from build123d import *

# Parameters (mm, degrees)
SKETCH1_R           = 1.016
SKETCH1_R_2         = 1.397
BOSS_EXTRUDE1_DEPTH = 3.175


with BuildPart() as part:
    # Sketch1 → Boss-Extrude1 (new body)
    with BuildSketch(Plane.XZ.offset(3.175)):
        with BuildLine():
            Line((12.7, 38.1), (6.35, 38.1))
            ThreePointArc((6.35, 38.1), (-7.120384182, 32.520384182), (-12.7, 19.05))
            Line((-12.7, 19.05), (-12.7, -38.1))
            Line((-12.7, -38.1), (12.7, -38.1))
            Line((12.7, -38.1), (12.7, 38.1))
        make_face()
        with Locations(Location((5.08, 20.828, 0), (0, 0, 90))):  # turned: the seam where the file's is
            Circle(SKETCH1_R, mode=Mode.SUBTRACT)
        with Locations(Location((-5.08, 20.828, 0), (0, 0, 90))):  # turned: the seam where the file's is
            Circle(SKETCH1_R, mode=Mode.SUBTRACT)
        with Locations(Location((-5.08, -27.792, 0), (0, 0, 90))):  # turned: the seam where the file's is
            Circle(SKETCH1_R, mode=Mode.SUBTRACT)
        with Locations(Location((5.08, -27.792, 0), (0, 0, 90))):  # turned: the seam where the file's is
            Circle(SKETCH1_R, mode=Mode.SUBTRACT)
        with Locations(Location((0, 31.75, 0), (0, 0, 90))):  # turned: the seam where the file's is
            Circle(SKETCH1_R_2, mode=Mode.SUBTRACT)
        Polygon((3.65, 17.018), (10, 17.018), (10, -23.982), (-10, -23.982), (-10, 17.018), (-3.65, 17.018), (-3.65, 20.193), (3.65, 20.193), align=None, mode=Mode.SUBTRACT)
    extrude(amount=-BOSS_EXTRUDE1_DEPTH)


solid = part.part
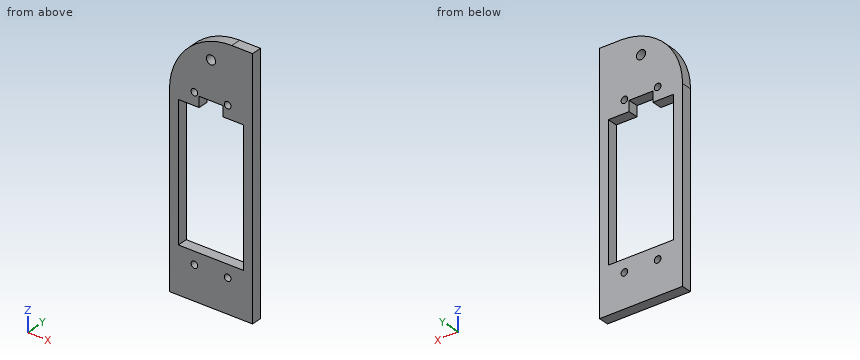
CAD build for the part. Positions are in the model's coordinates, mm. Round coordinates to 2 decimals unless told otherwise and drop trailing zeros. Write each loop counter-clockwise with the first axis right and the second up, starting at its lowest first coordinate (ties: lowest second). Pieces come first, ordered by that corner, then holes. Notation, with made-up numbers: M 83.5,84.25 L 89.5,84.25 A14 cw 89.5,100.25 Z; hole C -9,15 d4. An arc over 180 degrees is marked long. Use a Markdown table: item, result. Add a question column.
1. Slice it at B-B on x = -5.08. Give the cut face in (y, z) (3 decimals).
2. Slice it at A-A on z = -18. Give the cut face in (x, y) (3 decimals), then the cut area to 3 significant figures.
3. Slice it at D-D on x = -0.75. Give the cut face in (y, z) (3 decimals).
4. Flat gauge pins, fed straight in: P1, Ø1.8, axis at x = 5.08, z = -27.792, coming from the -Y side; P2, Ø2.5, axis at x = -5.08, z = 20.828, coming from the -Y side (3 decimals). Where does each tip first touch, or does it go through?
5. Slice it at C-C on y = -1.15. Give the cut face in (x, z), then the cut area to 3 significant figures.
6. Drill centre lines: probe 1 along X at (y, z) = (-0.55, 20.5); probe 2 along Z at (x, y) = (-5.08, -1.2); probe 3 along X at (y, z) = (-1.8, -23). Where is each one in solid material? Low to high.
Reply:
| question | item | result |
|---|---|---|
| 1 | outline | M -3.175,-38.1 L 0,-38.1 L 0,-28.808 L -3.175,-28.808 Z; M -3.175,-26.776 L 0,-26.776 L 0,-23.982 L -3.175,-23.982 Z; M -3.175,17.018 L 0,17.018 L 0,19.812 L -3.175,19.812 Z; M -3.175,21.844 L 0,21.844 L 0,34.29 L -3.175,34.29 Z |
| 2 | outline | M -12.7,-3.175 L -10,-3.175 L -10,0 L -12.7,0 Z; M 10,-3.175 L 12.7,-3.175 L 12.7,0 L 10,0 Z |
| 2 | area | 17.1 mm^2 |
| 3 | outline | M -3.175,-38.1 L 0,-38.1 L 0,-23.982 L -3.175,-23.982 Z; M -3.175,20.193 L 0,20.193 L 0,30.571 L -3.175,30.571 Z; M -3.175,32.929 L 0,32.929 L 0,36.727 L -3.175,36.727 Z |
| 4 | P1 | passes through |
| 4 | P2 | stops at y = -3.175 |
| 5 | outline | M -12.7,-38.1 L 12.7,-38.1 L 12.7,38.1 L 6.35,38.1 A19.05 ccw -12.7,19.05 Z; hole M -10,-23.98 L 10,-23.98 L 10,17.02 L 3.65,17.02 L 3.65,20.19 L -3.65,20.19 L -3.65,17.02 L -10,17.02 Z; hole C -5.08,-27.79 d2.03; hole C -5.08,20.83 d2.03; hole C 0,31.75 d2.79; hole C 5.08,-27.79 d2.03; hole C 5.08,20.83 d2.03 |
| 5 | area | 995 mm^2 |
| 6 | probe 1 | x = -12.64 to -6.04, -4.12 to 4.12, 6.04 to 12.7 |
| 6 | probe 2 | z = -38.1 to -28.81, -26.78 to -23.98, 17.02 to 19.81, 21.84 to 34.29 |
| 6 | probe 3 | x = -12.7 to -10, 10 to 12.7 |
